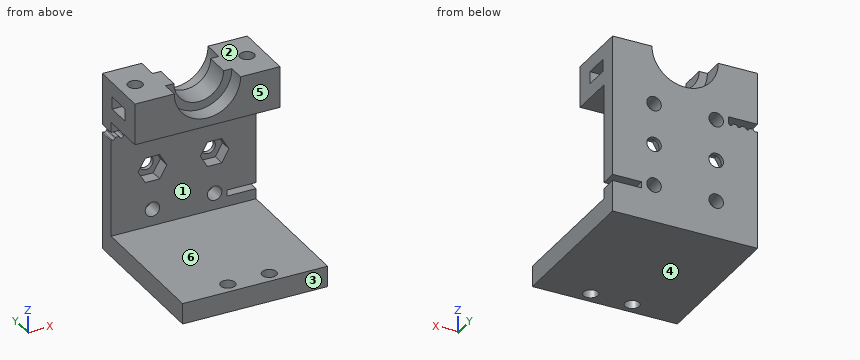
from build123d import *

# Parameters (mm, degrees)
SKETCH1_W           = 35
SKETCH1_H           = 28
BOSS_EXTRUDE1_DEPTH = 4
SKETCH2_R           = 1.75
CUT_EXTRUDE1_DEPTH  = 23.765104876
SKETCH3_W           = 35
SKETCH3_H           = 15
BOSS_EXTRUDE2_DEPTH = 10
CUT_REVOLVE1_ANGLE  = 180
SKETCH6_R           = 1.75
CUT_EXTRUDE3_DEPTH  = 10
SKETCH8_W           = 3
SKETCH8_H           = 6
CUT_EXTRUDE4_DEPTH  = 7
SKETCH9_W           = 3
SKETCH9_H           = 6
CUT_EXTRUDE5_DEPTH  = 7
SKETCH7_W           = 35
SKETCH7_H           = 37
BOSS_EXTRUDE3_DEPTH = 5
SKETCH10_R          = 1.75
CUT_EXTRUDE6_DEPTH  = 5
SKETCH18_W          = 7
SKETCH18_H          = 1.5
CUT_EXTRUDE14_DEPTH = 48.44733923
SKETCH19_R          = 1.75
CUT_EXTRUDE15_DEPTH = 48.44733923
CUT_EXTRUDE16_DEPTH = 3
SKETCH21_R          = 0.5
CUT_EXTRUDE17_DEPTH = 4
LPATTERN2_COUNT     = 4
LPATTERN2_PITCH     = 2
FILLET2_R           = 0.15


with BuildPart() as part:
    # Sketch1 → Boss-Extrude1 (new body)
    with BuildSketch(Plane(origin=(0, 0, 0), x_dir=(1, 0, 0), z_dir=(0, 1, 0))):
        Rectangle(SKETCH1_W, SKETCH1_H)
    extrude(amount=BOSS_EXTRUDE1_DEPTH)

    # Sketch2 → Cut-Extrude1 (cut, through all)
    with BuildSketch(Plane(origin=(0, 4, 0), x_dir=(1, 0, 0), z_dir=(0, 1, 0))):
        with Locations(Location((-7.5, -10, 0), (0, 0, 270))):
            Circle(SKETCH2_R)
        with Locations(Location((-7.5, 10, 0), (0, 0, 270))):
            Circle(SKETCH2_R)
        with Locations(Location((7.5, -10, 0), (0, 0, 270))):
            Circle(SKETCH2_R)
        with Locations(Location((7.5, 10, 0), (0, 0, 270))):
            Circle(SKETCH2_R)
    extrude(amount=-CUT_EXTRUDE1_DEPTH, mode=Mode.SUBTRACT)

    # Sketch3 → Boss-Extrude2 (add)
    with BuildSketch(Plane.XY.offset(14)):
        with Locations((0, -3.5)):
            Rectangle(SKETCH3_W, SKETCH3_H)
    extrude(amount=BOSS_EXTRUDE2_DEPTH)

    # Sketch5 → Cut-Revolve1 (revolve, cut)
    with BuildSketch(Plane.XY.offset(24)):
        Polygon((0, 4), (8, 4), (8, -1), (6, -1), (6, -7), (8, -7), (8, -11), (0, -11), align=None)
    revolve(axis=Axis((0, 4, 24), (0, 1, 0)), revolution_arc=CUT_REVOLVE1_ANGLE, mode=Mode.SUBTRACT)

    # Sketch6 → Cut-Extrude3 (cut)
    with BuildSketch(Plane.XY.offset(24)):
        with Locations((-13.5, -3.5)):
            Circle(SKETCH6_R)
        with Locations((13.5, -3.5)):
            Circle(SKETCH6_R)
    extrude(amount=-CUT_EXTRUDE3_DEPTH, mode=Mode.SUBTRACT)

    # Sketch8 → Cut-Extrude4 (cut)
    with BuildSketch(Plane.ZY.offset(17.5)):
        with Locations((19, -3.5)):
            Rectangle(SKETCH8_W, SKETCH8_H)
    extrude(amount=-CUT_EXTRUDE4_DEPTH, mode=Mode.SUBTRACT)

    # Sketch9 → Cut-Extrude5 (cut)
    with BuildSketch(Plane(origin=(17.5, 0, 0), x_dir=(0, 0, -1), z_dir=(1, 0, 0))):
        with Locations((-19, -3.5)):
            Rectangle(SKETCH9_W, SKETCH9_H)
    extrude(amount=-CUT_EXTRUDE5_DEPTH, mode=Mode.SUBTRACT)

    # Sketch7 → Boss-Extrude3 (add)
    with BuildSketch(Plane(origin=(0, 0, -14), x_dir=(-1, 0, 0), z_dir=(0, 0, -1))):
        with Locations((0, -14.5)):
            Rectangle(SKETCH7_W, SKETCH7_H)
    extrude(amount=BOSS_EXTRUDE3_DEPTH)

    # Sketch10 → Cut-Extrude6 (cut)
    with BuildSketch(Plane(origin=(0, 0, -19), x_dir=(-1, 0, 0), z_dir=(0, 0, -1))):
        with Locations((-5, -30)):
            Circle(SKETCH10_R)
        with Locations((5, -30)):
            Circle(SKETCH10_R)
    extrude(amount=-CUT_EXTRUDE6_DEPTH, mode=Mode.SUBTRACT)

    # Sketch18 → Cut-Extrude14 (cut, through all)
    with BuildSketch(Plane(origin=(0, 4, 0), x_dir=(1, 0, 0), z_dir=(0, 1, 0))):
        with Locations((-14, -10.75)):
            Rectangle(SKETCH18_W, SKETCH18_H)
        with Locations((14, 10.75)):
            Rectangle(SKETCH18_W, SKETCH18_H)
    extrude(amount=-CUT_EXTRUDE14_DEPTH, mode=Mode.SUBTRACT)

    # Sketch19 → Cut-Extrude15 (cut, through all)
    with BuildSketch(Plane(origin=(0, 4, 0), x_dir=(1, 0, 0), z_dir=(0, 1, 0))):
        with Locations(Location((-7.5, 0, 0), (0, 0, 270))):
            Circle(SKETCH19_R)
        with Locations(Location((7.5, 0, 0), (0, 0, 270))):
            Circle(SKETCH19_R)
    extrude(amount=-CUT_EXTRUDE15_DEPTH, mode=Mode.SUBTRACT)

    # Sketch20 → Cut-Extrude16 (cut)
    with BuildSketch(Plane.XZ):
        Polygon((10.964101615, 0), (9.232050808, 3), (5.767949192, 3), (4.035898385, 0), (5.767949192, -3), (9.232050808, -3), align=None)
        Polygon((-10.964101615, 0), (-9.232050808, -3), (-5.767949192, -3), (-4.035898385, 0), (-5.767949192, 3), (-9.232050808, 3), align=None)
    extrude(amount=-CUT_EXTRUDE16_DEPTH, mode=Mode.SUBTRACT)

    # Sketch21 → Cut-Extrude17 (cut)
    with BuildSketch(Plane(origin=(0, 4, 0), x_dir=(1, 0, 0), z_dir=(0, 1, 0))):
        with Locations((-17, -10)):
            Circle(SKETCH21_R)
    cut_extrude17 = extrude(amount=-CUT_EXTRUDE17_DEPTH, mode=Mode.SUBTRACT)

    # LPattern2: Cut-Extrude17 ×4
    with Locations(*[(i * LPATTERN2_PITCH, 0, 0) for i in range(1, LPATTERN2_COUNT)]):
        add(cut_extrude17, mode=Mode.SUBTRACT)

    # Fillet2
    fillet2_edges = [part.edges().sort_by_distance(p)[0] for p in [
        (-17.5, 2, 10),
        (-16.5, 2, 10),
        (-12.5, 2, 10),
        (-13.5, 2, 10),
        (-14.5, 2, 10),
        (-15.5, 2, 10),
        (-11.5, 2, 10),
    ]]
    fillet(fillet2_edges, radius=FILLET2_R)


solid = part.part
Read the model definition and answer for the solid it produces. Units are mm, in the model's axes. Face numbers are marked on the shaded views. A direction names the side the tool comes from. Give positions to 0.01 mm unless a question says otherwise; leave off trailing zeros. Write each loop counter-clockwise with the first axis right and the second up, starting at its lowest first coordinate (ties: lowest second). Pieces come first, ordered by that corner, then holes. Notation, with made-up numbers: (13, -12.75) -> (72, -12.75) arc R9 cw to (72, 1.25) -> close; hole circle Ø7 at (-6.5, 64.5). An arc over 180 degrees is marked (long way). Answer as a JSON object with one key per item and string values. Group by question number.
1) Find section A-A (y = -10). Write down the section's boundary in (x, z), and give its area (3 significant figures).
2) Find section B-B (x = 0). Write down the section's boundary in (y, z), and give its area (3 significant figures).
3) Find section D-D (y = -4.5). Count the separate pieces of the cut face and the enclosed holes in it, and give its area (3 significant figures).
4) Consider L1, parallel to Z at x = -15.5, y = -1; L2, parallel to Z at x = -8.5, y = -4; L3, parallel to Z at x = -4, y = -16.5. Determine where each line is inside the solid, lowest interval first. Write a range as from..to.
5) A tool of negligible diameter and unlimited length cuts with its end or side. For the marked faces 4, 5 and 6, from which of +Z, -Z, +X, -X, +Y, -Y can it reach the whole face along a straight path? Write none if from no direction.
6) The mould has two halves that part along Z. Classify the marked faces 1, 2 and 3: +Z half, -Z half, draft (parallel to the pull), parting line (faces both ways), or undercut.
7) Each of these flat-tipped pins is pushed along its axis until it touches: P1, Ø8, axis at x = 11, z = 12.5, coming from the -Y side; P2, Ø1, axis at x = -3, y = -26.5, coming from the +Z side; P3, Ø3, axis at x = 5, y = -30, coming from the -Z side; P4, Ø5, axis at x = 9, z = 0.5, coming from the -Y side. Where does it stop, or does it pass through?
8) Find section C-C (y = -30). Write down the section's boundary in (x, z), and give its area (3 significant figures).
Values follow:
{
 "1": {"outline": "(-17.5, -19) -> (17.5, -19) -> (17.5, -14) -> (-17.5, -14) -> close; (-17.5, 14) -> (17.5, 14) -> (17.5, 24) -> (8, 24) arc R8 cw to (-8, 24) -> (-17.5, 24) -> close", "area": "424 mm2"},
 "2": {"outline": "(-33, -19) -> (4, -19) -> (4, 16) -> (-1, 16) -> (-1, 18) -> (-7, 18) -> (-7, 16) -> (-11, 16) -> (-11, 14) -> (0, 14) -> (0, -14) -> (-33, -14) -> close", "area": "339 mm2"},
 "3": {"separate pieces": "6", "enclosed holes": "0", "area": "386 mm2"},
 "4": {"L1": "z = -19..-14, 14..17.5, 20.5..24", "L2": "z = -19..-14, 14..24", "L3": "z = -19..-14"},
 "5": {"face 4": "-Z, +X, -X, +Y, -Y", "face 5": "+Z, +X, -X, -Y", "face 6": "+X, -X, -Y"},
 "6": {"face 1": "undercut", "face 2": "+Z half", "face 3": "draft"},
 "7": {"P1": "stops at y = -11", "P2": "stops at z = -14", "P3": "passes through", "P4": "stops at y = 0"},
 "8": {"outline": "(-17.5, -19) -> (-6.75, -19) -> (-6.75, -14) -> (-17.5, -14) -> close; (-3.25, -19) -> (3.25, -19) -> (3.25, -14) -> (-3.25, -14) -> close; (6.75, -19) -> (17.5, -19) -> (17.5, -14) -> (6.75, -14) -> close", "area": "140 mm2"}
}
